Can you work these out from the model? Positions are in its coordinate system, mm. Round coordinates to 2 decimals unless told otherwise and drop trailing zeros. Loops run counter-clockwise (first coordinate to the right, second up) from the corner with the lowest first, then second, coordinate; pieces in that order, holes last.
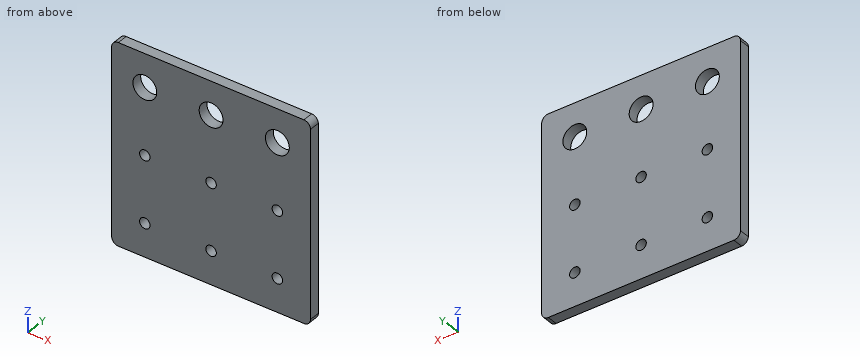
```python
from build123d import *

# Parameters (mm, degrees)
F0_W     = 150
F0_H     = 150
F0_R     = 3.95
F0_R_2   = 9
F1_DEPTH = 8
F2_R     = 5
F3_R     = 5
F4_R     = 5
F5_R     = 5


with BuildPart() as f1:
    # F0 (on Front) → F1 (new body)
    with BuildSketch(Plane.XZ):
        Rectangle(F0_W, F0_H)
        with Locations((-50, -50)):
            Circle(F0_R, mode=Mode.SUBTRACT)
        with Locations((0, -50)):
            Circle(F0_R, mode=Mode.SUBTRACT)
        with Locations((50, -50)):
            Circle(F0_R, mode=Mode.SUBTRACT)
        with Locations((-50, 0)):
            Circle(F0_R, mode=Mode.SUBTRACT)
        with Locations((-50, 50)):
            Circle(F0_R_2, mode=Mode.SUBTRACT)
        Circle(F0_R, mode=Mode.SUBTRACT)
        with Locations((50, 0)):
            Circle(F0_R, mode=Mode.SUBTRACT)
        with Locations((0, 50)):
            Circle(F0_R_2, mode=Mode.SUBTRACT)
        with Locations((50, 50)):
            Circle(F0_R_2, mode=Mode.SUBTRACT)
    extrude(amount=F1_DEPTH)

    # F2
    f2_edges = [f1.edges().sort_by_distance(p)[0] for p in [
        (75, -4, 75),
    ]]
    fillet(f2_edges, radius=F2_R)

    # F3
    f3_edges = [f1.edges().sort_by_distance(p)[0] for p in [
        (75, -4, -75),
    ]]
    fillet(f3_edges, radius=F3_R)

    # F4
    f4_edges = [f1.edges().sort_by_distance(p)[0] for p in [
        (-75, -4, -75),
    ]]
    fillet(f4_edges, radius=F4_R)

    # F5
    f5_edges = [f1.edges().sort_by_distance(p)[0] for p in [
        (-75, -4, 75),
    ]]
    fillet(f5_edges, radius=F5_R)


solid = f1.part
```
(1) Suppose I cut it at B-B (x = -50). Write out the boundary of the cut face in (y, z), then the cut area to 3 significant figures.
(2) If I drill on line 1 (Z direction, x = 0, y = -5); line 2 (X direction, y = -6, z = 52.5); line 3 (X direction, y = -6.75, z = 50.5), over which ranges is the centre line in solid material (lowest first)?
(3) Suppose I cut it at A-A (z = 0). Write out the boundary of the cut face in (x, y).
(4) Suppose I cut it at D-D (x = 56.5). Write out the boundary of the cut face in (y, z), then the cut area to 3 significant figures.
(5) Suppose I cut it at C-C (y = -2.5). Give the number of separate pieces and of enclosed holes in the cut face, then the cut area to 3 significant figures.
Check result:
1. outline: (-8, -75) - (0, -75) - (0, -53.95) - (-8, -53.95) - close; (-8, -46.05) - (0, -46.05) - (0, -3.95) - (-8, -3.95) - close; (-8, 3.95) - (0, 3.95) - (0, 41) - (-8, 41) - close; (-8, 59) - (0, 59) - (0, 75) - (-8, 75) - close
1. area: 930 mm2
2. line 1: z = -75 to -53.95, -46.05 to -3.95, 3.95 to 41, 59 to 75
2. line 2: x = -75 to -58.65, -41.35 to -8.65, 8.65 to 41.35, 58.65 to 75
2. line 3: x = -75 to -58.99, -41.01 to -8.99, 8.99 to 41.01, 58.99 to 75
3. outline: (-75, -8) - (-53.95, -8) - (-53.95, 0) - (-75, 0) - close; (-46.05, -8) - (-3.95, -8) - (-3.95, 0) - (-46.05, 0) - close; (3.95, -8) - (46.05, -8) - (46.05, 0) - (3.95, 0) - close; (53.95, -8) - (75, -8) - (75, 0) - (53.95, 0) - close
4. outline: (-8, -75) - (0, -75) - (0, 43.78) - (-8, 43.78) - close; (-8, 56.22) - (0, 56.22) - (0, 75) - (-8, 75) - close
4. area: 1,100 mm2
5. separate pieces: 1
5. enclosed holes: 9
5. area: 21,400 mm2
